Here's how the part is built. I have some questions about the finished solid (model axes, mm). A direction names the side the tool comes from. Coordinates: 2 decimals unless noted, no trailing zeros. Write each loop counter-clockwise with the first axis right and the second up, starting at its lowest first coordinate (ties: lowest second). Pieces come first, ordered by that corner, then holes.
Item 1: For faces 4 (the face through (22.749, 18.564, -35.692)), 5 (the face through (22.269, -17.19, -29.612)), 6 (the face through (25.4, -16, 1)), which set-ups out of +Z, -Z, +X, -X, +Y, -Y let a thin tool reach every point of the face, with its end or its side?
Item 2: Please list where these lines run through material, in increasing order: line 1 (Z direction, x = 40.15, y = 0) (3 decimals); line 2 (Z direction, x = 38.35, y = 0) (3 decimals); line 3 (Y direction, x = 31.5, z = -10.5).
Item 3: I want a section at C-C (x = 21). Please give me the cut outline in (y, z).
Item 4: If we mould it in two halves opening along Z, with no side actions, what happens to faces 1 (the face through (44.45, -6.2, -2)), 2 (the face through (22.54, -1.38, -6.2)), 3 (the face through (21.509, -8.755, -39.427))? For each: pulls with the +Z half, pulls with the -Z half, needs draft (parallel to the pull), parting line crosses it, or undercut.
Item 5: I'm going to push flat-ended pins straight in: P1, Ø10, axis at x = 13.5, y = 7.5, coming from the -Z side; P2, Ø1.5, axis at x = 20, z = 3, coming from the -Y side; P3, Ø2, axis at x = 30.5, z = -37, coming from the +Y side. Where does each tip first touch, or does it pass through?
Item 6: I want a section at D-D (z = 0). Count the separate pieces of the cut face and the enclosed holes in it, and give its area (3 significant figures).
Item 7: I want a section at B-B (x = 5.5). Please give me the cut outline in (y, z) (3 decimals), and give its area (3 significant figures).
from build123d import *

# Parameters (mm, degrees)
F2_R     = 6.35
F3_DEPTH = 76.2
F5_DEPTH = 41.276


with BuildPart() as f1:
    # F0 (on Top) → F1 (revolve)
    with BuildSketch(Plane.XY):
        Polygon((0, 9.525), (0, 0), (22.225, 0), (44.45, 0), (44.45, 9.525), (25.4, 13.086654), (25.4, 36.349638), (37.581098, 47.625), (41.275, 47.625), (41.275, 50.8), (33.009252, 50.8), (22.225, 39.692349), (10.784252, 50.8), (3.175, 50.8), (3.175, 47.625), (6.868902, 47.625), (19.05, 36.349638), (19.05, 13.086654), align=None)
    revolve(axis=Axis((22.225, 0, 0), (1, 0, 0)))

    # F2 (on face) → F3 (cut)
    with BuildSketch(Plane.YZ.offset(44.45)):
        Circle(F2_R)
    extrude(amount=-F3_DEPTH, mode=Mode.SUBTRACT)

    # F4 (on face) → F5 (cut, through all)
    with BuildSketch(Plane.YZ.offset(41.275)):
        with BuildLine():
            ThreePointArc((-12.80801, 31.942442), (-17.109062, 29.659415), (-21.236747, 27.076108))
            Line((-21.236747, 27.076108), (-8.941196, 11.399711))
            ThreePointArc((-8.941196, 11.399711), (-7.569379, 13.189774), (-5.315075, 13.255492))
            Line((-5.315075, 13.255492), (-12.80801, 31.942442))
        make_face()
        with BuildLine():
            Line((34.066971, 4.853508), (14.343037, 2.043447))
            ThreePointArc((14.343037, 2.043447), (15.207368, -0.039612), (14.13713, -2.024756))
            Line((14.13713, -2.024756), (34.066971, -4.879159))
            ThreePointArc((34.066971, -4.879159), (34.240338, -0.012825), (34.066971, 4.853508))
        make_face()
        with BuildLine():
            ThreePointArc((-21.258962, -27.063283), (-17.131276, -29.646589), (-12.830224, -31.929617))
            Line((-12.830224, -31.929617), (-5.401842, -13.443158))
            ThreePointArc((-5.401842, -13.443158), (-7.63799, -13.150161), (-8.822055, -11.230736))
            Line((-8.822055, -11.230736), (-21.258962, -27.063283))
        make_face()
    extrude(amount=-F5_DEPTH, mode=Mode.SUBTRACT)


solid = f1.part
Answer:
1. face 4: none
1. face 5: +X, -X
1. face 6: +X
2. line 1: z = -50.8 to -47.625, -10.329 to -6.35, 6.35 to 10.329, 47.625 to 50.8
2. line 2: z = -50.8 to -47.625, -10.665 to -6.35, 6.35 to 10.665, 47.625 to 50.8
2. line 3: y = -48.11 to -40.66, -5.7 to 5.7, 40.66 to 48.11
3. outline: circle Ø81.76 at (0, 0); hole (-21.26, -27.06) arc R68.39 ccw to (-12.83, -31.93) - (-5.4, -13.44) arc R2.63 cw to (-8.82, -11.23) - close; hole (-21.24, 27.08) - (-8.94, 11.4) arc R2.63 cw to (-5.32, 13.26) - (-12.81, 31.94) arc R68.38 ccw to start; hole circle Ø12.7 at (0, 0); hole (14.14, -2.02) - (34.07, -4.88) arc R68.38 ccw to (34.07, 4.85) - (14.34, 2.04) arc R2.63 cw to start
4. face 1: needs draft
4. face 2: undercut
4. face 3: parting line crosses it
5. P1: stops at z = -50.69
5. P2: stops at y = -42.48
5. P3: stops at y = 32.86
6. separate pieces: 3
6. enclosed holes: 0
6. area: 1,050 mm2
7. outline: circle Ø101.6 at (0, 0); circle Ø21.107 at (0, 0); hole circle Ø95.25 at (0, 0); hole circle Ø12.7 at (0, 0)
7. area: 1,200 mm2
